Verification items for the finished model (mm, model axes). Give positions to 0.01 mm unless a question says otherwise; leave off trailing zeros. Order: outer loops, then holes, each group sorted by start corner. A loop starts at its lowest first (then second) coordinate and runs counter-clockwise, first axis right, second up. Notation, with made-up numbers: (38, 1.5) -> (92, 1.5) arc R35 cw to (92, 40.5) -> close; hole circle Ø7 at (55, 52.5). An arc over 180 degrees is marked (long way). Return JSON: item names as keys, results as strings. Group by question number.
(1) Thickness scan on line 1 along Z through (x, y) = (-75, -1.5); line 2 along Z through (x, y) = (-62.5, -0.5); line 3 along X through (y, z) = (1, 115). Record the ranges inside material, lowest first.
(2) Cross-section at B-B on y = 2.5. State how many separate pieces and enclosed holes the cut face has, then the cut area to 3 significant figures.
(3) Cross-section at C-C on x = -96. Enter the section's corners in (y, z), then the cut area to 3 significant figures.
(4) Cross-section at D-D on z = -4. Enter the section's corners in (x, y).
(5) Cross-section at A-A on z = -115. Enter the section's corners in (x, y).
(6) Depth check by flat-ended pin: pin 1 Ø3 at (x, z) = (64, -26) entering from +Y; pin 2 Ø1 at (y, z) = (-3, -116) entering from -X. Enter the tip coordinate at first touch or a pass-through.
from build123d import *

# Parameters (mm, degrees)
SKETCH_1_R         = 3.25
SKETCH_1_R_2       = 37.5
SKETCH_1_R_3       = 2.25
SKETCH_1_R_4       = 1.75
EXTRUDE_1639_DEPTH = 4
FILLET_1_R         = 10
HOLE_WIZARD_3_5_D  = 3.5


with BuildPart() as part:
    # Эскиз1 → Extrude 1639 (new, symmetric)
    with BuildSketch(Plane(origin=(0, 0, 0), x_dir=(1, 0, 0), z_dir=(0, 1, 0))):
        Polygon((273.664027596, -136.63804004), (18.5, 305.31902002), (-18.5, 305.31902002), (-273.664027596, -136.63804004), (-255.164027596, -168.68097998), (255.164027596, -168.68097998), align=None)
        with Locations(Location((-250.557621135, -144.65951001, 0), (0, 0, 270))):
            Circle(SKETCH_1_R, mode=Mode.SUBTRACT)
        with Locations(Location((250.557621135, -144.65951001, 0), (0, 0, 270))):
            Circle(SKETCH_1_R, mode=Mode.SUBTRACT)
        with Locations(Location((0, 289.31902002, 0), (0, 0, 270))):
            Circle(SKETCH_1_R, mode=Mode.SUBTRACT)
        with Locations(Location((0, 115, 0), (0, 0, 270))):
            Circle(SKETCH_1_R_2, mode=Mode.SUBTRACT)
        with Locations(Location((36, 151, 0), (0, 0, 270))):
            Circle(SKETCH_1_R_3, mode=Mode.SUBTRACT)
        with Locations(Location((-36, 151, 0), (0, 0, 270))):
            Circle(SKETCH_1_R_3, mode=Mode.SUBTRACT)
        with Locations(Location((-36, 79, 0), (0, 0, 270))):
            Circle(SKETCH_1_R_3, mode=Mode.SUBTRACT)
        with Locations(Location((36, 79, 0), (0, 0, 270))):
            Circle(SKETCH_1_R_3, mode=Mode.SUBTRACT)
        with Locations(Location((-64, 57, 0), (0, 0, 270))):
            Circle(SKETCH_1_R_4, mode=Mode.SUBTRACT)
        with Locations(Location((-64, -10, 0), (0, 0, 270))):
            Circle(SKETCH_1_R_4, mode=Mode.SUBTRACT)
        with Locations(Location((64, -10, 0), (0, 0, 270))):
            Circle(SKETCH_1_R_4, mode=Mode.SUBTRACT)
        with Locations(Location((64, 26, 0), (0, 0, 270))):
            Circle(SKETCH_1_R_4, mode=Mode.SUBTRACT)
        with Locations(Location((75, -65, 0), (0, 0, 270))):
            Circle(SKETCH_1_R_4, mode=Mode.SUBTRACT)
        with Locations(Location((75, -115, 0), (0, 0, 270))):
            Circle(SKETCH_1_R_4, mode=Mode.SUBTRACT)
        with Locations(Location((-75, -115, 0), (0, 0, 270))):
            Circle(SKETCH_1_R_4, mode=Mode.SUBTRACT)
        with Locations(Location((-75, -65, 0), (0, 0, 270))):
            Circle(SKETCH_1_R_4, mode=Mode.SUBTRACT)
    extrude(amount=EXTRUDE_1639_DEPTH, both=True)

    # Скругление1
    fillet_1_edges = [part.edges().sort_by_distance(p)[0] for p in [
        (255.164027596, 0, 168.68097998),
        (-255.164027596, 0, 168.68097998),
        (-273.664027596, 0, 136.63804004),
        (-18.5, 0, -305.31902002),
        (18.5, 0, -305.31902002),
        (273.664027596, 0, 136.63804004),
    ]]
    fillet(fillet_1_edges, radius=FILLET_1_R)

    # К Профилю 3,5мм (through all)
    with Locations(Plane(origin=(0, 4, 0), x_dir=(1, 0, 0), z_dir=(0, 1, 0))):
        with Locations((-137.42175976, 79.34048999), (-62.42175976, 209.244300558), (62.42175976, 209.244300558), (137.42175976, 79.34048999), (212.42175976, -50.563320578), (150, -158.68097998), (0, -158.68097998), (-150, -158.68097998), (-212.42175976, -50.563320578)):
            Hole(HOLE_WIZARD_3_5_D / 2)


solid = part.part
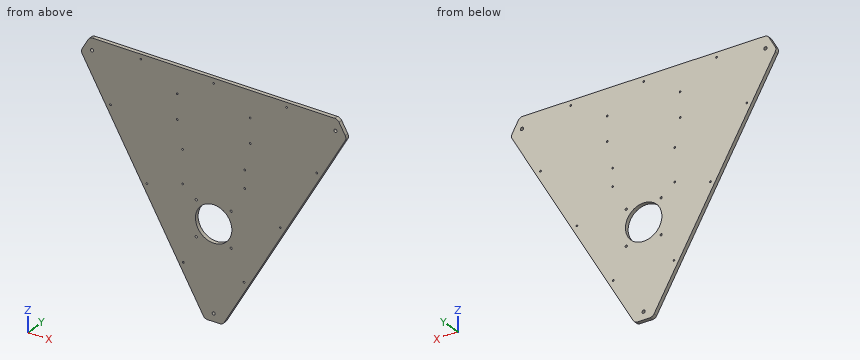
Verdict:
{
 "1": {"line 1": "-207.46 to 63.25, 66.75 to 113.25, 116.75 to 168.68", "line 2": "-229.11 to -210.99, -207.5 to -57.9, -56.1 to 9.1, 10.9 to 168.68", "line 3": "-261.17 to -76.75, -73.25 to 73.25, 76.75 to 261.17"},
 "2": {"separate pieces": "1", "enclosed holes": "25", "area": "141,000 mm²"},
 "3": {"outline": "(-4, -171.09) -> (4, -171.09) -> (4, 168.68) -> (-4, 168.68) -> close", "area": "2,720 mm²"},
 "4": {"outline": "(-192.47, -4) -> (192.47, -4) -> (192.47, 4) -> (-192.47, 4) -> close"},
 "5": {"outline": "(-128.38, -4) -> (-37.5, -4) -> (-37.5, 4) -> (-128.38, 4) -> close; (37.5, -4) -> (128.38, -4) -> (128.38, 4) -> (37.5, 4) -> close"},
 "6": {"pin 1": "through", "pin 2": "x = -128.09"}
}
